from build123d import *

# Parameters (mm, degrees)
F0_R     = 3
F0_R_2   = 2.5
F1_DEPTH = 507
F2_R     = 2
F3_R     = 7


# Not quite as in the source:
# - a feature names something its author has since deleted; it is built from what else it names


with BuildPart() as f1:
    # F0 (on Top) → F1 (new body)
    with BuildSketch(Plane.XY):
        with BuildLine():
            Line((18.15, -30), (30, -30))
            Line((30, -30), (30, -18.15))
            Line((30, -18.15), (27.5, -18.15))
            Line((27.5, -18.15), (27.5, -20.15))
            Line((27.5, -20.15), (21.5477069044, -20.15))
            ThreePointArc((21.5477069044, -20.15), (19.5, -15), (21.5477069044, -9.85))
            Line((21.5477069044, -9.85), (27.5, -9.85))
            Line((27.5, -9.85), (27.5, -11.85))
            Line((27.5, -11.85), (30, -11.85))
            Line((30, -11.85), (30, 11.85))
            Line((30, 11.85), (27.5, 11.85))
            Line((27.5, 11.85), (27.5, 9.85))
            Line((27.5, 9.85), (21.5477069044, 9.85))
            ThreePointArc((21.5477069044, 9.85), (19.5, 15), (21.5477069044, 20.15))
            Line((21.5477069044, 20.15), (27.5, 20.15))
            Line((27.5, 20.15), (27.5, 18.15))
            Line((27.5, 18.15), (30, 18.15))
            Line((30, 18.15), (30, 30))
            Line((30, 30), (18.15, 30))
            Line((18.15, 30), (18.15, 27.5))
            Line((18.15, 27.5), (20.15, 27.5))
            Line((20.15, 27.5), (20.15, 21.5477069044))
            ThreePointArc((20.15, 21.5477069044), (15, 19.5), (9.85, 21.5477069044))
            Line((9.85, 21.5477069044), (9.85, 27.5))
            Line((9.85, 27.5), (11.85, 27.5))
            Line((11.85, 27.5), (11.85, 30))
            Line((11.85, 30), (-11.85, 30))
            Line((-11.85, 30), (-11.85, 27.5))
            Line((-11.85, 27.5), (-9.85, 27.5))
            Line((-9.85, 27.5), (-9.85, 21.5477069044))
            ThreePointArc((-9.85, 21.5477069044), (-15, 19.5), (-20.15, 21.5477069044))
            Line((-20.15, 21.5477069044), (-20.15, 27.5))
            Line((-20.15, 27.5), (-18.15, 27.5))
            Line((-18.15, 27.5), (-18.15, 30))
            Line((-18.15, 30), (-30, 30))
            Line((-30, 30), (-30, 18.15))
            Line((-30, 18.15), (-27.5, 18.15))
            Line((-27.5, 18.15), (-27.5, 20.15))
            Line((-27.5, 20.15), (-21.5477069044, 20.15))
            ThreePointArc((-21.5477069044, 20.15), (-19.5, 15), (-21.5477069044, 9.85))
            Line((-21.5477069044, 9.85), (-27.5, 9.85))
            Line((-27.5, 9.85), (-27.5, 11.85))
            Line((-27.5, 11.85), (-30, 11.85))
            Line((-30, 11.85), (-30, -11.85))
            Line((-30, -11.85), (-27.5, -11.85))
            Line((-27.5, -11.85), (-27.5, -9.85))
            Line((-27.5, -9.85), (-21.5477069044, -9.85))
            ThreePointArc((-21.5477069044, -9.85), (-19.5, -15), (-21.5477069044, -20.15))
            Line((-21.5477069044, -20.15), (-27.5, -20.15))
            Line((-27.5, -20.15), (-27.5, -18.15))
            Line((-27.5, -18.15), (-30, -18.15))
            Line((-30, -18.15), (-30, -30))
            Line((-30, -30), (-18.15, -30))
            Line((-18.15, -30), (-18.15, -27.5))
            Line((-18.15, -27.5), (-20.15, -27.5))
            Line((-20.15, -27.5), (-20.15, -21.5477069044))
            ThreePointArc((-20.15, -21.5477069044), (-15, -19.5), (-9.85, -21.5477069044))
            Line((-9.85, -21.5477069044), (-9.85, -27.5))
            Line((-9.85, -27.5), (-11.85, -27.5))
            Line((-11.85, -27.5), (-11.85, -30))
            Line((-11.85, -30), (11.85, -30))
            Line((11.85, -30), (11.85, -27.5))
            Line((11.85, -27.5), (9.85, -27.5))
            Line((9.85, -27.5), (9.85, -21.5477069044))
            ThreePointArc((9.85, -21.5477069044), (15, -19.5), (20.15, -21.5477069044))
            Line((20.15, -21.5477069044), (20.15, -27.5))
            Line((20.15, -27.5), (18.15, -27.5))
            Line((18.15, -27.5), (18.15, -30))
        make_face()
        with Locations((-25, -25)):
            Circle(F0_R, mode=Mode.SUBTRACT)
        with Locations((-15, -15)):
            Circle(F0_R_2, mode=Mode.SUBTRACT)
        with Locations((25, -25)):
            Circle(F0_R, mode=Mode.SUBTRACT)
        with Locations((15, -15)):
            Circle(F0_R_2, mode=Mode.SUBTRACT)
        with Locations((-25, 25)):
            Circle(F0_R, mode=Mode.SUBTRACT)
        with Locations((-15, 15)):
            Circle(F0_R_2, mode=Mode.SUBTRACT)
        Polygon((-7, 22), (-7, 27.5), (0, 27.5), (7, 27.5), (7, 22), (10, 16), (10, 10), (16, 10), (22, 7), (27.5, 7), (27.5, 0), (27.5, -7), (22, -7), (16, -10), (10, -10), (10, -16), (7, -22), (7, -27.5), (0, -27.5), (-7, -27.5), (-7, -22), (-10, -16), (-10, -10), (-16, -10), (-22, -7), (-27.5, -7), (-27.5, 0), (-27.5, 7), (-22, 7), (-16, 10), (-10, 10), (-10, 16), align=None, mode=Mode.SUBTRACT)
        with Locations((15, 15)):
            Circle(F0_R_2, mode=Mode.SUBTRACT)
        with Locations((25, 25)):
            Circle(F0_R, mode=Mode.SUBTRACT)
    extrude(amount=F1_DEPTH)

    # F2
    f2_edges = [f1.edges().sort_by_distance(p)[0] for p in [
        (-7, 27.5, 253.5),
        (7, 27.5, 253.5),
    ]]
    fillet(f2_edges, radius=F2_R)

    # F3
    f3_edges = [f1.edges().sort_by_distance(p)[0] for p in [
        (-10, 16, 253.5),
        (10, 16, 253.5),
    ]]
    fillet(f3_edges, radius=F3_R)


solid = f1.part
Work out the finished part from the listing and answer in its coordinate system (mm). A direction names the side the tool comes from. Give positions to 0.01 mm unless a question says otherwise; leave off trailing zeros. Use a Markdown table: item, result. Add a question column.
1) For a pull along X with two mould halves and no side action, classify faces 3 (the cylindrical face through (19.5, -15.1, 250)), 4 (the flat face through (30, -24, 250)), 5 (the flat face through (-30, -24, 250)) as +X half, -X half, draft (parallel to the pull), parting line (faces both ways), or undercut.
2) Consider line 1 along X through (y, z) = (5, 68.5); line 2 along Y through (x, z) = (14.5, 219); line 3 along Y through (x, z) = (15, 267). Determine where each line is inside the solid, lowest interval first.
3) Each of these flat-tipped pins is pushed along its axis until it touches: P1, Ø6.5, axis at x = 15, y = 15, coming from the +Z side; P2, Ø5.5, axis at x = 25, y = -25, coming from the +Z side. Where does it stop, or does it pass through?
4) Which of the six approach directions +Z, -Z, +X, -X, +Y, -Y give full straight-line access (tool end or side, diameter ignored) to faces 1 (the cylindrical face through (15.1, 19.5, 250)), 2 (the flat face through (0, 30, 250))?
5) The part is cut by section A-A, the plane z = 296. Count the separate pieces of the cut face and the enclosed holes in it, plus the area to 3 significant figures.
Reported:
| question | item | result |
|---|---|---|
| 1 | face 3 | undercut |
| 1 | face 4 | +X half |
| 1 | face 5 | -X half |
| 2 | line 1 | x = -30 to -27.5, 27.5 to 30 |
| 2 | line 2 | y = -19.52 to -17.45, -12.55 to -10, 10 to 12.55, 17.45 to 19.52 |
| 2 | line 3 | y = -19.5 to -17.5, -12.5 to -10, 10 to 12.5, 17.5 to 19.5 |
| 3 | P1 | stops at z = 507 |
| 3 | P2 | passes through |
| 4 | face 1 | +Z, -Z |
| 4 | face 2 | +Z, -Z, +X, -X, +Y |
| 5 | separate pieces | 1 |
| 5 | enclosed holes | 9 |
| 5 | area | 1,080 mm^2 |
